Geometry: see drawing. Coordinates: mm, zero at the bounding-box minimum. A direction names the side the tool comes from. Give positions to 0.01 mm unless a question says otherwise; leave off trailing zeros. Write each loop counter-clockwise with the first axis right and the second up, starting at its lowest first coordinate (ties: lowest second). Pieces come first, ordered by that corner, then holes.
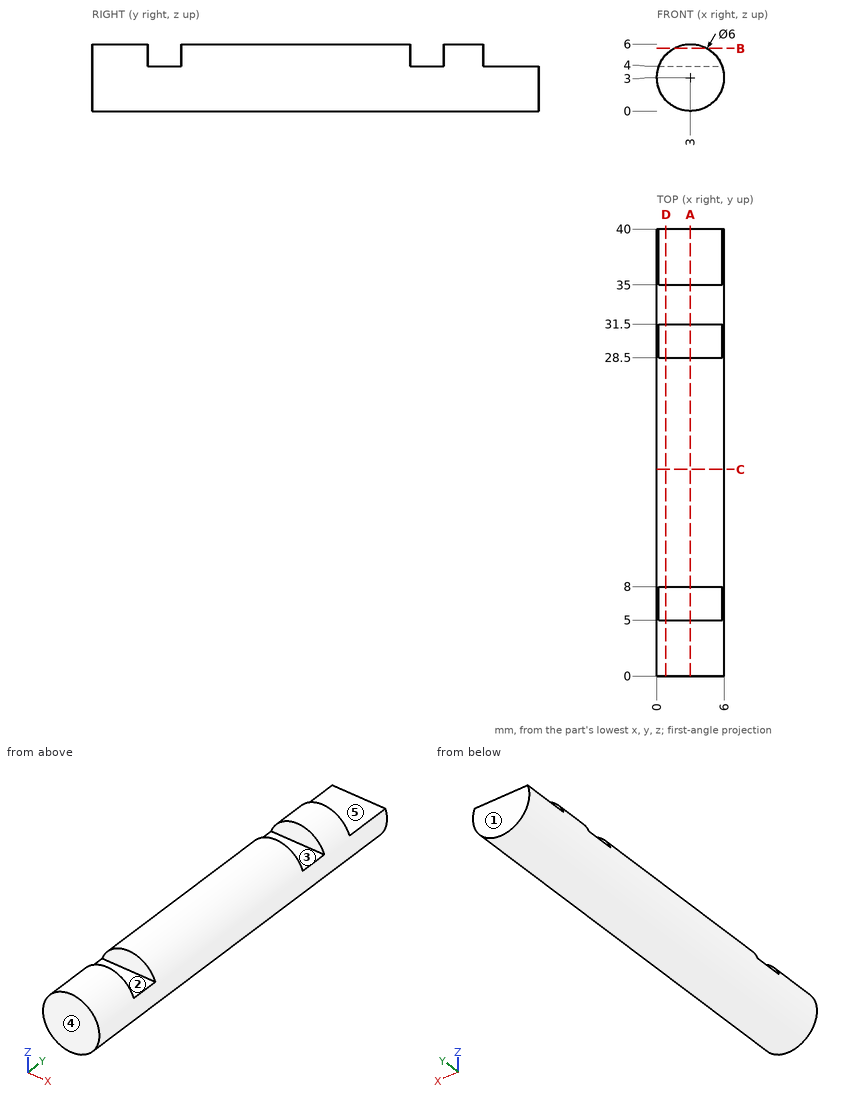
Q1. Section C-C, the plane y = 18.5. Return the cut outline in (x, z).
Q2. Section B-B, the plane z = 5.6. Return the cut outline in (x, y).
Q3. Pin query (flat end, axial travel): pin 1 (1.6 mm diameter, centred on x = 2.5, z = 5.5, fed in from +Y); pin 2 (0.9 mm diameter, centred on x = 4, y = 6, fed in from +Z). Return the tip coordinate at first contact, or that it passes through.
Q4. Mould query, pull axis Y, two halves, no side actions, for the marked faces 3, 4 and 5. Classes: +Y half, -Y half, draft (parallel to the pull), parting line (faces both ways), or undercut.
Q5. Section D-D, the plane x = 0.8. Return the cut outline in (y, z).
Q6. Material intervals for line 1 along Y through (x, z) = (2.65, 5.2); line 2 along Z through (x, y) = (2.95, 29.5); line 3 along X through (y, z) = (23, 1.3), sorted ascending.
Q7. Section A-A, the plane x = 3. Return the cut outline in (y, z).
Q8. Access query for the marked faces 1 and 2. Directions: +Z, -Z, +X, -X, +Y, -Y. A direction counts if a zero-diameter tool reaches every point of the face in a straight line with its end or side. Return the directions, or none.
Solutions:
1. outline: circle Ø6 at (3, 3)
2. outline: (1.5, 0) - (4.5, 0) - (4.5, 5) - (1.5, 5) - close; (1.5, 8) - (4.5, 8) - (4.5, 28.5) - (1.5, 28.5) - close; (1.5, 31.5) - (4.5, 31.5) - (4.5, 35) - (1.5, 35) - close
3. pin 1: stops at y = 35
3. pin 2: stops at z = 4
4. face 3: undercut
4. face 4: -Y half
4. face 5: draft
5. outline: (0, 0.96) - (40, 0.96) - (40, 4) - (35, 4) - (35, 5.04) - (31.5, 5.04) - (31.5, 4) - (28.5, 4) - (28.5, 5.04) - (8, 5.04) - (8, 4) - (5, 4) - (5, 5.04) - (0, 5.04) - close
6. line 1: y = 0 to 5, 8 to 28.5, 31.5 to 35
6. line 2: z = 0 to 4
6. line 3: x = 0.53 to 5.47
7. outline: (0, 0) - (40, 0) - (40, 4) - (35, 4) - (35, 6) - (31.5, 6) - (31.5, 4) - (28.5, 4) - (28.5, 6) - (8, 6) - (8, 4) - (5, 4) - (5, 6) - (0, 6) - close
8. face 1: +Z, -Z, +X, -X, +Y
8. face 2: +Z, +X, -X
